The model under review builds one solid part; all positions refer to its coordinate system, in mm. Coordinates: 2 decimals unless noted, no trailing zeros. Order: outer loops, then holes, each group sorted by start corner. A loop starts at its lowest first (then second) coordinate and runs counter-clockwise, first axis right, second up. Notation, with made-up numbers: M 71,3.25 L 123,3.25 A26 ccw 123,20.25 Z; hole C 79,66 d4. An arc over 180 degrees is marked long. Answer in a Markdown table with one row per item.
from build123d import *

# Parameters (mm, degrees)
SKETCH1_R           = 5
BOSS_EXTRUDE1_DEPTH = 27
FILLET1_R           = 2
SKETCH2_W           = 3
SKETCH2_H           = 1.5
BOSS_EXTRUDE2_DEPTH = 3
SKETCH3_R           = 0.75
CUT_EXTRUDE1_DEPTH  = 5


with BuildPart() as part:
    # Sketch1 → Boss-Extrude1 (new body)
    with BuildSketch(Plane.XY):
        Circle(SKETCH1_R)
    extrude(amount=BOSS_EXTRUDE1_DEPTH)

    # Fillet1
    fillet1_edges = [part.edges().sort_by_distance(p)[0] for p in [
        (-5, 0, 27),
    ]]
    fillet(fillet1_edges, radius=FILLET1_R)

    # Sketch2 → Boss-Extrude2 (add)
    with BuildSketch(Plane(origin=(0, 0, 0), x_dir=(-1, 0, 0), z_dir=(0, 0, -1))):
        Rectangle(SKETCH2_W, SKETCH2_H)
    extrude(amount=BOSS_EXTRUDE2_DEPTH)

    # Sketch3 → Cut-Extrude1 (cut)
    with BuildSketch(Plane(origin=(0, 0.75, 0), x_dir=(1, 0, 0), z_dir=(0, 1, 0))):
        with Locations(Location((0, 1.5, 0), (0, 0, 270))):
            Circle(SKETCH3_R)
    extrude(amount=-CUT_EXTRUDE1_DEPTH, mode=Mode.SUBTRACT)


solid = part.part
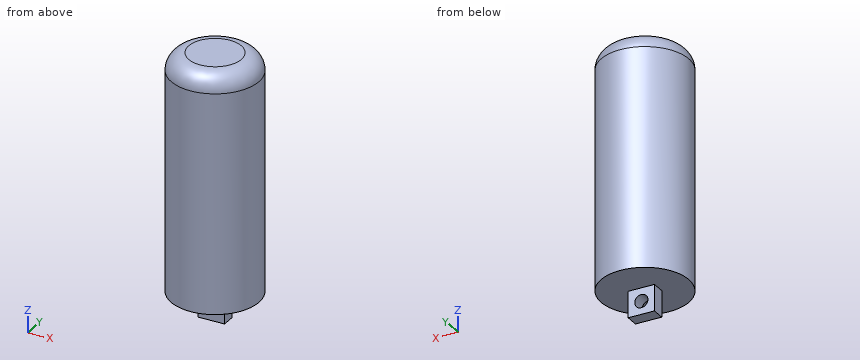
(1) Take a section at B-B (x = 0). Write out the cut boundary in (y, z).
Report:
| item | result |
|---|---|
| outline | M -5,0 L -0.75,0 L -0.75,-0.75 L 0.75,-0.75 L 0.75,0 L 5,0 L 5,25 A2 ccw 3,27 L -3,27 A2 ccw -5,25 Z; M -0.75,-3 L 0.75,-3 L 0.75,-2.25 L -0.75,-2.25 Z |
(2) Insertion check: P1, Ø1.5, axis at x = 0, z = -2, coming from the -Y side; P2, Ø2, axis at x = -2.5, z = 8, coming from the -Y side; P3, Ø5, axis at x = -1.5, y = 2.5, coming from the -Z side; P4, Ø2, axis at x = 0, z = -1.5, coming from the +Y side. Each pin has a flat end and moves straight along its axis. Give the tip position at first contact, or say it passes through.
Report:
| item | result |
|---|---|
| P1 | y = -0.75 |
| P2 | y = -4.77 |
| P3 | z = -3 |
| P4 | y = 0.75 |
(3) Take a section at C-C (y = 0). Write out the cut boundary in (x, z).
Report:
| item | result |
|---|---|
| outline | M -5,0 L -1.5,0 L -1.5,-3 L 1.5,-3 L 1.5,0 L 5,0 L 5,25 A2 ccw 3,27 L -3,27 A2 ccw -5,25 Z; hole C 0,-1.5 d1.5 |
(4) Take a section at A-A (z = -1.5). Write out the cut boundary in (x, y).
Report:
| item | result |
|---|---|
| outline | M -1.5,-0.75 L -0.75,-0.75 L -0.75,0.75 L -1.5,0.75 Z; M 0.75,-0.75 L 1.5,-0.75 L 1.5,0.75 L 0.75,0.75 Z |
(5) Take a section at D-D (z = 7.5). Write out the cut boundary in (x, y), then the cut area to 3 significant figures.
Report:
| item | result |
|---|---|
| outline | C 0,0 d10 |
| area | 78.5 mm^2 |
(6) To check wall thickness, follow line 1 (X direction, y = -0.1, z = -1.5); line 2 (Y direction, x = -4, z = 5.5); line 3 (Y direction, x = 2.25, z = 23). State the ranges of each line that lie inside material, in increasing order. Write a range as [from, to].
Report:
| item | result |
|---|---|
| line 1 | [-1.5, -0.75], [0.75, 1.5] |
| line 2 | [-3, 3] |
| line 3 | [-4.47, 4.47] |
